```python
from build123d import *

# Parameters (mm, degrees)
CUT_EXTRUDE1_DEPTH  = 87.011627121
CIRPATTERN1_COUNT   = 3
BOSS_EXTRUDE1_DEPTH = 1
CIRPATTERN2_COUNT   = 3
SKETCH4_R           = 1.65
CUT_EXTRUDE2_DEPTH  = 86.334635407
CIRPATTERN3_COUNT   = 6
SKETCH5_R           = 5.95
CUT_EXTRUDE3_DEPTH  = 84.054199171


with BuildPart() as part:
    # Sketch1 → Revolve1 (revolve)
    with BuildSketch(Plane.XY, mode=Mode.PRIVATE) as revolve1_sk:
        Polygon((50.5, 19), (50.5, 14), (57, 14), (57, -14), (26, -14), (26, -11), (16, -11), (16, -8), (27.242640687, -8), (30.242640687, -11), (52, -11), (52, 5.428932188), (38.428932188, 19), align=None)
    revolve(revolve1_sk.sketch.rotate(Axis((0, 34.277777778, 0), (0, -1, 0)), 90), axis=Axis((0, 34.277777778, 0), (0, -1, 0)))

    # Sketch2 → Cut-Extrude1 (cut, through all)
    with BuildSketch(Plane(origin=(0, -11, 0), x_dir=(1, 0, 0), z_dir=(0, 1, 0))):
        with BuildLine():
            Line((20, 53.37602458), (12.98245614, 34.647594903))
            ThreePointArc((12.98245614, 34.647594903), (32.04293994, 18.5), (36.496925436, -6.08066063))
            Line((36.496925436, -6.08066063), (56.22499324, -9.367504214))
            ThreePointArc((56.22499324, -9.367504214), (49.363448016, 28.5), (20, 53.37602458))
        make_face()
    cut_extrude1 = extrude(amount=CUT_EXTRUDE1_DEPTH, mode=Mode.SUBTRACT)

    # CirPattern1: Cut-Extrude1 ×3 about axis
    cirpattern1_axis = Axis((0, 0, 0), (0, 1, 0))
    for i in range(1, CIRPATTERN1_COUNT):
        add(cut_extrude1.rotate(cirpattern1_axis, i * 360 / CIRPATTERN1_COUNT), mode=Mode.SUBTRACT)

    # Sketch3 → Boss-Extrude1 (add)
    with BuildSketch(Plane(origin=(0, 19, 0), x_dir=(1, 0, 0), z_dir=(0, 1, 0))):
        with BuildLine():
            ThreePointArc((10.273190717, 46.339368728), (0, 47.464466094), (-10.273190717, 46.339368728))
            ThreePointArc((-10.273190717, 46.339368728), (-12.552759897, 42.761161865), (-8.974553034, 40.481592685))
            ThreePointArc((-8.974553034, 40.481592685), (0, 41.464466094), (8.974553034, 40.481592685))
            ThreePointArc((8.974553034, 40.481592685), (12.552759897, 42.761161865), (10.273190717, 46.339368728))
        make_face()
    boss_extrude1 = extrude(amount=BOSS_EXTRUDE1_DEPTH)

    # CirPattern2: Boss-Extrude1 ×3 about axis
    cirpattern2_axis = Axis((0, 0, 0), (0, 1, 0))
    for i in range(1, CIRPATTERN2_COUNT):
        add(boss_extrude1.rotate(cirpattern2_axis, i * 360 / CIRPATTERN2_COUNT))

    # Sketch4 → Cut-Extrude2 (cut, through all)
    with BuildSketch(Plane(origin=(0, -8, 0), x_dir=(1, 0, 0), z_dir=(0, 1, 0))):
        with Locations(Location((20, 0, 0), (0, 0, 270))):
            Circle(SKETCH4_R)
    cut_extrude2 = extrude(amount=-CUT_EXTRUDE2_DEPTH, mode=Mode.SUBTRACT)

    # CirPattern3: Cut-Extrude2 ×6 about axis
    cirpattern3_axis = Axis((0, 0, 0), (0, 1, 0))
    for i in range(1, CIRPATTERN3_COUNT):
        add(cut_extrude2.rotate(cirpattern3_axis, i * 360 / CIRPATTERN3_COUNT), mode=Mode.SUBTRACT)

    # Sketch5 → Cut-Extrude3 (cut, through all)
    with BuildSketch(Plane.XY):
        with Locations(Location((0, 0, 0), (0, 0, 65.842722295))):
            Circle(SKETCH5_R)
    extrude(amount=-CUT_EXTRUDE3_DEPTH, mode=Mode.SUBTRACT)


solid = part.part
```
For this review, take the finished solid that the model builds, in its own axes (mm). A direction names the side the tool comes from. Give positions to 0.01 mm unless a question says otherwise; leave off trailing zeros. Write each loop counter-clockwise with the first axis right and the second up, starting at its lowest first coordinate (ties: lowest second). Pieces come first, ordered by that corner, then holes.
Item 1: The part is to be moulded in two halves that separate along X. For faces 6 (the face through (-32.48, 7.26, 39.46)), 7 (the face through (0, 20, -44)), 8 (the face through (-41.178, 19.493, 23.607)), say which applies: +X half, -X half, draft (parallel to the pull), parting line (faces both ways), or undercut.
Item 2: Insertion check: P1, Ø12, axis at x = -28, y = 13.5, coming from the -Z side; P2, Ø3, axis at x = -16, y = 6.5, coming from the +Z side; P3, Ø4, axis at x = 10, z = 17.32, coming from the -Y side; P4, Ø3, axis at x = -20, z = 0, coming from the -Y side. Each pin has a flat end and moves straight along its axis. Give the tip position at first contact, or say it passes through.
Item 3: Wall thickness on probe 1 along Y at (x, z) = (-50, -12); probe 2 along X at (y, z) = (-10.5, -3); probe 3 along X at (y, z) = (-2, 18): over which ranges is each line inside the solid? List them lowest first.
Item 4: Machinability: for faces 1 (the face through (15.821, -12.479, -20.633)), 2 (the face through (-0.3, -6.3, -52)), 3 (the face through (-0.3, 16.5, -50.5)), 4 (the face through (0, 19, -40)), 5 (the face through (45, 14, 26)), which of the approach directions +Z, -Z, +X, -X, +Y, -Y give a long, thin tool a straight path to every point of the face, cutting with its end or side? Answer none if there is none.
Item 5: Take a section at C-C (x = 0). Give the boundary of the cut face in (y, z).
Item 6: Take a section at D-D (y = 8). Give the boundary of the cut face in (x, z) (1 decimal), and give its area (3 significant figures).
Item 7: Take a section at A-A (z = 0). Give the boundary of the cut face in (x, y), and give its area (3 significant figures).
Item 8: Take a section at B-B (y = 1). Give the boundary of the cut face in (x, z) (1 decimal).
Established:
1. face 6: undercut
1. face 7: draft
1. face 8: -X half
2. P1: stops at z = 23.07
2. P2: stops at z = -46.68
2. P3: stops at y = -11
2. P4: passes through
3. probe 1: y = -14 to -11
3. probe 2: x = -29.59 to -15.72, 15.72 to 29.59
3. probe 3: x = -54.08 to -48.79, 48.79 to 54.08
4. face 1: -Y
4. face 2: none
4. face 3: -Z, +Y
4. face 4: +Y
4. face 5: +Z, +X, +Y
5. outline: (-14, -57) - (-5.95, -57) - (-5.95, -52) - (-11, -52) - (-11, -30.24) - (-8, -27.24) - (-8, -16) - (-11, -16) - (-11, -26) - (-14, -26) - close; (-14, 26) - (-11, 26) - (-11, 16) - (-8, 16) - (-8, 27.24) - (-11, 30.24) - (-11, 57) - (-14, 57) - close; (5.95, -57) - (14, -57) - (14, -50.5) - (19, -50.5) - (19, -47.46) - (20, -47.46) - (20, -41.46) - (19, -41.46) - (19, -38.43) - (5.95, -51.48) - close
6. outline: (-56.2, 9.4) - (-48.8, 8.1) arc R49.4 cw to (-31.4, 38.2) - (-36.2, 44) arc R57 ccw to start; (-20, -53.4) arc R57 ccw to (20, -53.4) - (17.3, -46.3) arc R49.4 cw to (-17.3, -46.3) - close; (31.4, 38.2) arc R49.4 cw to (48.8, 8.1) - (56.2, 9.4) arc R57 ccw to (36.2, 44) - close
6. area: 867 mm2
7. outline: (-57, -14) - (-26, -14) - (-26, -11) - (-21.65, -11) - (-21.65, -8) - (-27.24, -8) - (-30.24, -11) - (-57, -11) - close; (-18.35, -11) - (-16, -11) - (-16, -8) - (-18.35, -8) - close; (16, -11) - (18.35, -11) - (18.35, -8) - (16, -8) - close; (21.65, -11) - (26, -11) - (26, -14) - (57, -14) - (57, -11) - (30.24, -11) - (27.24, -8) - (21.65, -8) - close
7. area: 243 mm2
8. outline: (-56.2, 9.4) - (-51.3, 8.5) arc R52 cw to (-33, 40.1) - (-36.2, 44) arc R57 ccw to start; (-20, -53.4) arc R57 ccw to (-5.9, -56.7) - (-5.9, -51.7) arc R52 cw to (-18.2, -48.7) - close; (5.9, -56.7) arc R57 ccw to (20, -53.4) - (18.2, -48.7) arc R52 cw to (5.9, -51.7) - close; (33, 40.1) arc R52 cw to (51.3, 8.5) - (56.2, 9.4) arc R57 ccw to (36.2, 44) - close
